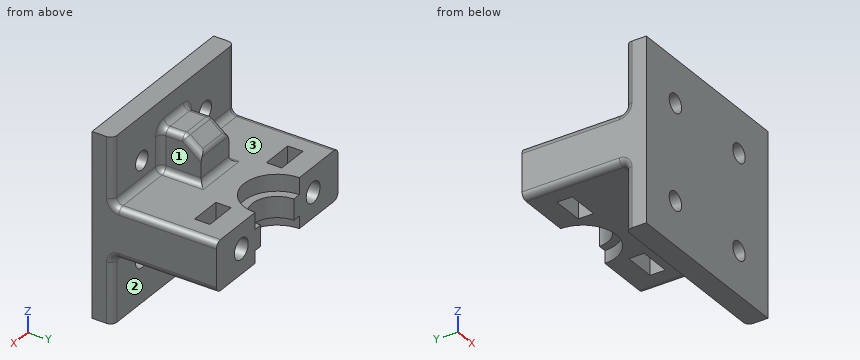
```python
from build123d import *

# Parameters (mm, degrees)
SKETCH1_W           = 44
SKETCH1_H           = 44
BOSS_EXTRUDE1_DEPTH = 5
SKETCH2_W           = 44
SKETCH2_H           = 12
BOSS_EXTRUDE2_DEPTH = 25
SKETCH3_R           = 2.5
CUT_EXTRUDE1_DEPTH  = 15
SKETCH4_W           = 7.7
SKETCH4_H           = 3.7
CUT_EXTRUDE2_DEPTH  = 29
SKETCH6_R           = 8
CUT_EXTRUDE3_DEPTH  = 4
CUT_EXTRUDE4_DEPTH  = 3
BOSS_EXTRUDE3_DEPTH = 5
SKETCH10_R          = 2.25
CUT_EXTRUDE5_DEPTH  = 10
FILLET2_R           = 1.5


with BuildPart() as part:
    # Sketch1 → Boss-Extrude1 (new body)
    with BuildSketch(Plane(origin=(0, 0, 0), x_dir=(1, 0, 0), z_dir=(0, 1, 0))):
        with Locations((22, 22)):
            Rectangle(SKETCH1_W, SKETCH1_H)
    extrude(amount=BOSS_EXTRUDE1_DEPTH)

    # Sketch2 → Boss-Extrude2 (add)
    with BuildSketch(Plane(origin=(0, 5, 0), x_dir=(1, 0, 0), z_dir=(0, 1, 0))):
        with Locations((22, 22)):
            Rectangle(SKETCH2_W, SKETCH2_H)
    extrude(amount=BOSS_EXTRUDE2_DEPTH)

    # Sketch3 → Cut-Extrude1 (cut)
    with BuildSketch(Plane(origin=(0, 30, 0), x_dir=(1, 0, 0), z_dir=(0, 1, 0))):
        with Locations((35, 22)):
            Circle(SKETCH3_R)
        with Locations((9, 22)):
            Circle(SKETCH3_R)
    extrude(amount=-CUT_EXTRUDE1_DEPTH, mode=Mode.SUBTRACT)

    # Sketch4 → Cut-Extrude2 (cut, through all)
    with BuildSketch(Plane.XY.offset(-16)):
        with Locations((9, 23.15)):
            Rectangle(SKETCH4_W, SKETCH4_H)
        with BuildLine():
            Line((16, 30), (28, 30))
            ThreePointArc((28, 30), (22, 36), (16, 30))
        make_face()
        with BuildLine():
            ThreePointArc((16, 30), (22, 24), (28, 30))
            Line((28, 30), (16, 30))
        make_face()
        with Locations((35, 23.15)):
            Rectangle(SKETCH4_W, SKETCH4_H)
    extrude(amount=-CUT_EXTRUDE2_DEPTH, mode=Mode.SUBTRACT)

    # Sketch6 → Cut-Extrude3 (cut)
    with BuildSketch(Plane.XY.offset(-16)):
        with Locations((22, 30)):
            Circle(SKETCH6_R)
    extrude(amount=-CUT_EXTRUDE3_DEPTH, mode=Mode.SUBTRACT)

    # Sketch7 → Cut-Extrude4 (cut)
    with BuildSketch(Plane(origin=(0, 0, -28), x_dir=(-1, 0, 0), z_dir=(0, 0, -1))):
        with BuildLine():
            Line((-30, 30), (-14, 30))
            ThreePointArc((-14, 30), (-22, 22), (-30, 30))
        make_face()
    extrude(amount=-CUT_EXTRUDE4_DEPTH, mode=Mode.SUBTRACT)

    # Sketch8 → Boss-Extrude3 (add, symmetric)
    with BuildSketch(Plane(origin=(22, 0, 0), x_dir=(0, 0, -1), z_dir=(1, 0, 0))):
        Polygon((16, 5), (6, 5), (6, 11), (9, 15), (16, 15), align=None)
    extrude(amount=BOSS_EXTRUDE3_DEPTH, both=True)

    # Sketch10 → Cut-Extrude5 (cut)
    with BuildSketch(Plane(origin=(0, 5, 0), x_dir=(1, 0, 0), z_dir=(0, 1, 0))):
        with Locations((33.5, 10.5)):
            Circle(SKETCH10_R)
        with Locations((10.5, 10.5)):
            Circle(SKETCH10_R)
        with Locations((33.5, 33.5)):
            Circle(SKETCH10_R)
        with Locations((10.5, 33.5)):
            Circle(SKETCH10_R)
    extrude(amount=-CUT_EXTRUDE5_DEPTH, mode=Mode.SUBTRACT)

    # Fillet2
    fillet2_edges = [part.edges().sort_by_distance(p)[0] for p in [
        (44, 5, -8),
        (35.5, 5, -16),
        (17, 10, -16),
        (22, 15, -16),
        (17, 13, -7.5),
        (22, 15, -9),
        (17, 8, -6),
        (22, 11, -6),
        (17, 5, -11),
        (22, 5, -6),
        (27, 10, -16),
        (27, 13, -7.5),
        (27, 8, -6),
        (27, 5, -11),
        (0, 5, -8),
        (44, 5, -36),
        (0, 17.5, -28),
        (8.5, 5, -16),
        (0, 17.5, -16),
        (44, 17.5, -16),
        (22, 5, -28),
        (44, 17.5, -28),
        (0, 5, -36),
    ]]
    fillet(fillet2_edges, radius=FILLET2_R)


solid = part.part
```
For this review, take the finished solid that the model builds, in its own axes (mm). Face numbers are marked on the shaded views. A direction names the side the tool comes from. Round coordinates to 2 decimals unless told otherwise and drop trailing zeros. Write each loop counter-clockwise with the first axis right and the second up, starting at its lowest first coordinate (ties: lowest second). Pieces come first, ordered by that corner, then holes. Notation, with made-up numbers: (20, -21.5) - (32, -21.5) arc R19 cw to (32, -6.5) - close; hole circle Ø2 at (-35.75, 31.5). An arc over 180 degrees is marked (long way). Write each question's results on one line, items separated by ' | '.
Item 1: For pin 1 (4 mm diameter, centred on x = 36, z = -38, fed in from -Y); pin 2 (2.5 mm diameter, centred on x = 34.5, z = -22.5, fed in from +Y); pin 3 (4.5 mm diameter, centred on x = 28.5, z = -6, fed in from +Y); pin 4 (8 mm diameter, centred on x = 27, y = 23, fed in from +Z), all flat-tipped, find the tip position at first contact; note any pin that passes through.
Calculated:
pin 1: stops at y = 0 | pin 2: stops at y = 15 | pin 3: stops at y = 11.81 | pin 4: stops at z = -16
Item 2: For the marked faces 1, 2 and 3, list the 3-axis set-ups (+Z, -Z, +X, -X, +Y, -Y) from which the entire face can be reached by the end or side of a thin tool; tool diameter is ignored.
Calculated:
face 1: +Z, +X, +Y | face 2: -Z, +X, -X, +Y | face 3: +Z, +Y
Item 3: Take a section at A-A on x = 10.5. Count the separate pieces of the cut face and the enclosed holes in it, then the cut area to 3 significant figures.
Calculated:
separate pieces: 5 | enclosed holes: 0 | area: 386 mm^2
Item 4: Take a section at C-C on y = 8.5. State the section outline as (x, z) points, then the cut area to 3 significant figures.
Calculated:
outline: (0, -26.5) arc R1.5 ccw to (1.5, -28) - (42.5, -28) arc R1.5 ccw to (44, -26.5) - (44, -17.5) arc R1.5 ccw to (42.5, -16) - (28.5, -16) arc R1.5 cw to (27, -14.5) - (27, -7.5) arc R1.5 ccw to (25.5, -6) - (18.5, -6) arc R1.5 ccw to (17, -7.5) - (17, -14.5) arc R1.5 cw to (15.5, -16) - (1.5, -16) arc R1.5 ccw to (0, -17.5) - close | area: 626 mm^2
Item 5: Take a section at B-B on y = 19.5. State the section outline as (x, z) points, then the cut area to 3 significant figures.
Calculated:
outline: (0, -26.5) arc R1.5 ccw to (1.5, -28) - (42.5, -28) arc R1.5 ccw to (44, -26.5) - (44, -17.5) arc R1.5 ccw to (42.5, -16) - (1.5, -16) arc R1.5 ccw to (0, -17.5) - close; hole circle Ø5 at (9, -22); hole circle Ø5 at (35, -22) | area: 487 mm^2
Item 6: To check wall thickness, follow line 1 along Z through (x, y) = (10.5, 2.55); line 2 along X through (y, z) = (3.6, -10.5); line 3 along X through (y, z) = (26.75, -23.5). State the ranges of each line that lie inside material, in increasing order. Write a range as from..to.
Calculated:
line 1: z = -44..-35.75, -31.25..-12.75, -8.25..0 | line 2: x = 0..8.25, 12.75..31.25, 35.75..44 | line 3: x = 0..7, 11..16.96, 27.04..33, 37..44
